Input: part model. Units: mm. Frame: model coordinates. Face numbers are marked on the shaded views. Coordinates: 2 decimals unless noted, no trailing zeros. Write each loop counter-clockwise with the first axis right and the second up, starting at its lowest first coordinate (ties: lowest second). Pieces come first, ordered by that corner, then holes. Notation, with made-up numbers: (48.25, 49.5) - (54.25, 49.5) arc R22 ccw to (54.25, 81.5) - close; hole circle Ø10 at (-15.5, 4). An arc over 180 degrees is marked (long way). One line per question, with ' | ' between items. Start each with the question number.
1) First-contact query: P1, Ø2.5, axis at x = 139.93, y = 0.92, coming from the -Z side; P2, Ø4, axis at x = 164.87, y = -0.92, coming from the +Z side. Flat tips, straight axial feed; report the tip coordinate or a pass-through.
2) Line query: line 1 (X direction, y = -7, z = 275.75); line 2 (X direction, y = 34, z = 274); line 3 (Y direction, x = 140, z = 273) (3 decimals). Output: solid intervals per line, ascending.
3) Section query C-C on y = 53.7. Return loops of the section in (x, z).
4) Section query D-D on z = 274.5. Give the number of separate pieces and of enclosed holes in the cut face, and give its area (3 significant figures).
5) Draft query along X for the marked faces 1, 2 and 3. Return one class per face: released by +X, released by -X, zero draft, split by the parting line, or undercut.
6) Section query A-A on x = 134.4. Return loops of the section in (y, z) (3 decimals), and give its area (3 significant figures).
7) Section query B-B on x = 152.4. Return loops of the section in (y, z) (3 decimals), and give its area (3 significant figures).
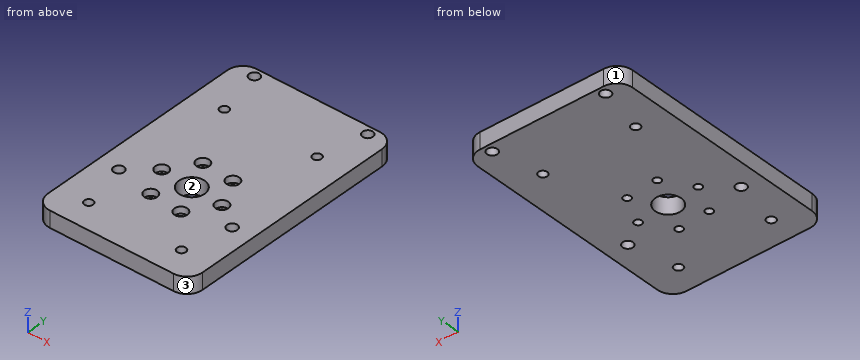
```python
from build123d import *

# Parameters (mm, degrees)
DISCO_1_4IN_START                     = 269.6
DISCO_1_4IN_DEPTH                     = 6.35
BARRENOS_M4_ESCUADRAS_PASADORES_START = 269.6
CROQUIS14_R                           = 1.45
CROQUIS14_R_2                         = 5
CROQUIS14_R_3                         = 1.25
CROQUIS14_R_4                         = 2
BARRENOS_M4_ESCUADRAS_PASADORES_DEPTH = 6.35
REFRENTADO_M2_5_START                 = 273.35
CROQUIS15_R                           = 2.5
REFRENTADO_M2_5_DEPTH                 = 2.6
PASO_M3_ESCUADRAS_TUERCA_START        = 269.6
CROQUIS16_R                           = 1.7
PASO_M3_ESCUADRAS_TUERCA_DEPTH        = 6.35


with BuildPart() as part:
    # Croquis13 → Disco_1-4in (new body)
    with BuildSketch(Plane.XY.offset(DISCO_1_4IN_START)):
        with BuildLine():
            Line((128.4, -36), (176.4, -36))
            ThreePointArc((176.4, -36), (180.642640687, -34.242640687), (182.4, -30))
            Line((182.4, -30), (182.4, 50.875))
            ThreePointArc((182.4, 50.875), (180.642640687, 55.117640687), (176.4, 56.875))
            Line((176.4, 56.875), (128.4, 56.875))
            ThreePointArc((128.4, 56.875), (124.157359313, 55.117640687), (122.4, 50.875))
            Line((122.4, 50.875), (122.4, -30))
            ThreePointArc((122.4, -30), (124.157359313, -34.242640687), (128.4, -36))
        make_face()
    extrude(amount=DISCO_1_4IN_DEPTH)

    # Croquis14 → Barrenos_M4_escuadras_pasadores (cut)
    with BuildSketch(Plane.XY.offset(BARRENOS_M4_ESCUADRAS_PASADORES_START)):
        with Locations((159.426042223, 10.338507178)):
            Circle(CROQUIS14_R)
        with Locations((146.959611258, 11.253984643)):
            Circle(CROQUIS14_R)
        with Locations((139.933569035, 0.915477464)):
            Circle(CROQUIS14_R)
        with Locations((145.373957777, -10.338507178)):
            Circle(CROQUIS14_R)
        with Locations((157.840388742, -11.253984643)):
            Circle(CROQUIS14_R)
        with Locations((164.866430965, -0.915477464)):
            Circle(CROQUIS14_R)
        with Locations((152.4, 0)):
            Circle(CROQUIS14_R_2)
        with Locations((134.4, 35.525)):
            Circle(CROQUIS14_R_3)
        with Locations((134.4, -25.525)):
            Circle(CROQUIS14_R_3)
        with Locations((170.4, 35.525)):
            Circle(CROQUIS14_R_3)
        with Locations((170.4, -25.525)):
            Circle(CROQUIS14_R_3)
        with Locations((130.4, 53.7)):
            Circle(CROQUIS14_R_4)
        with Locations((130.4, -7.35)):
            Circle(CROQUIS14_R_4)
        with Locations((174.4, 53.7)):
            Circle(CROQUIS14_R_4)
        with Locations((174.4, -7.35)):
            Circle(CROQUIS14_R_4)
    extrude(amount=BARRENOS_M4_ESCUADRAS_PASADORES_DEPTH, mode=Mode.SUBTRACT)

    # Croquis15 → Refrentado_M2-5 (cut)
    with BuildSketch(Plane.XY.offset(REFRENTADO_M2_5_START)):
        with Locations((159.426042223, 10.338507178)):
            Circle(CROQUIS15_R)
        with Locations((146.959611258, 11.253984643)):
            Circle(CROQUIS15_R)
        with Locations((139.933569035, 0.915477464)):
            Circle(CROQUIS15_R)
        with Locations((145.373957777, -10.338507178)):
            Circle(CROQUIS15_R)
        with Locations((157.840388742, -11.253984643)):
            Circle(CROQUIS15_R)
        with Locations((164.866430965, -0.915477464)):
            Circle(CROQUIS15_R)
    extrude(amount=REFRENTADO_M2_5_DEPTH, mode=Mode.SUBTRACT)

    # Croquis16 → Paso_M3_escuadras_tuerca (cut)
    with BuildSketch(Plane.XY.offset(PASO_M3_ESCUADRAS_TUERCA_START)):
        with Locations((134.4, 35.525)):
            Circle(CROQUIS16_R)
        with Locations((134.4, -25.525)):
            Circle(CROQUIS16_R)
        with Locations((170.4, 35.525)):
            Circle(CROQUIS16_R)
        with Locations((170.4, -25.525)):
            Circle(CROQUIS16_R)
    extrude(amount=PASO_M3_ESCUADRAS_TUERCA_DEPTH, mode=Mode.SUBTRACT)


solid = part.part
```
Answer key:
1) P1: through | P2: z = 273.35
2) line 1: 122.4 to 128.43, 132.37 to 172.43, 176.37 to 182.4 | line 2: 122.4 to 133.65, 135.15 to 169.65, 171.15 to 182.4 | line 3: -36 to -0.533, 2.364 to 56.875
3) outline: (123.11, 269.6) - (128.4, 269.6) - (128.4, 275.95) - (123.11, 275.95) - close; (132.4, 269.6) - (172.4, 269.6) - (172.4, 275.95) - (132.4, 275.95) - close; (176.4, 269.6) - (181.69, 269.6) - (181.69, 275.95) - (176.4, 275.95) - close
4) separate pieces: 1 | enclosed holes: 15 | area: 5,260 mm²
5) face 1: released by -X | face 2: undercut | face 3: released by +X
6) outline: (-36, 269.6) - (-27.225, 269.6) - (-27.225, 275.95) - (-36, 275.95) - close; (-23.825, 269.6) - (33.825, 269.6) - (33.825, 275.95) - (-23.825, 275.95) - close; (37.225, 269.6) - (56.875, 269.6) - (56.875, 275.95) - (37.225, 275.95) - close | area: 547 mm²
7) outline: (-36, 269.6) - (-5, 269.6) - (-5, 275.95) - (-36, 275.95) - close; (5, 269.6) - (56.875, 269.6) - (56.875, 275.95) - (5, 275.95) - close | area: 526 mm²
